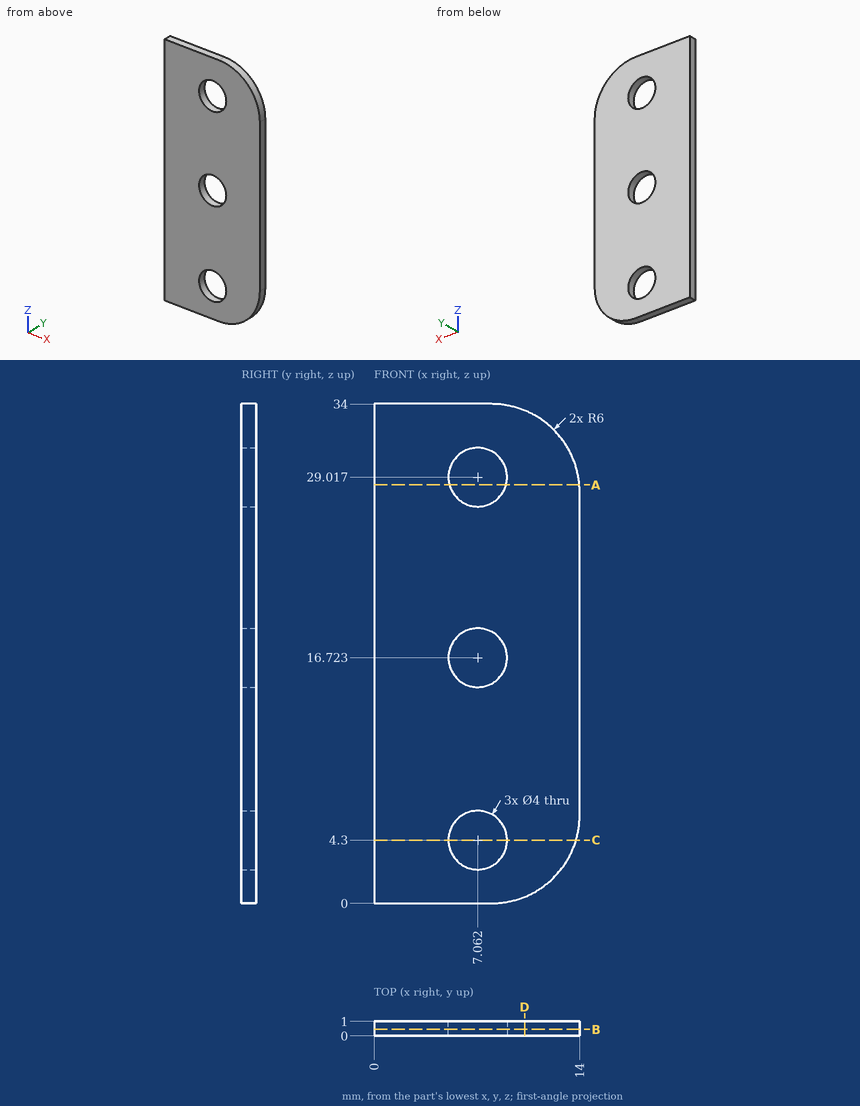
Drawing for the job (mm, zero at the part's lowest x, y, z). Round coordinates to 2 decimals unless told otherwise and drop trailing zeros. Loops run counter-clockwise (first coordinate to the right, second up) from the corner with the lowest first, then second, coordinate; pieces in that order, holes last.
1. Band-saw the part on B-B, the plane y = 0.45. List the corners of the cut face in (x, z), and give its area (3 significant figures).
Check values:
outline: (0, 0) - (8, 0) arc R6 ccw to (14, 6) - (14, 28) arc R6 ccw to (8, 34) - (0, 34) - close; hole circle Ø4 at (7.06, 4.3); hole circle Ø4 at (7.06, 16.72); hole circle Ø4 at (7.06, 29.02)
area: 423 mm2
2. Wall check: probe 1 along Z at (x, y) = (7, 0.8) (1 decimal); probe 2 along X at (y, z) = (0.7, 29) (1 decimal); probe 3 along X at (y, z) = (0.3, 18.5) (1 decimal). Give the ranges that are in metal, low to high.
Check values:
probe 1: z = 0 to 2.3, 6.3 to 14.7, 18.7 to 27, 31 to 34
probe 2: x = 0 to 5.1, 9.1 to 13.9
probe 3: x = 0 to 6.1, 8 to 14
3. Band-saw the part on D-D, the plane x = 10.25. List the corners of the cut face in (y, z).
Check values:
outline: (0, 0.44) - (1, 0.44) - (1, 33.56) - (0, 33.56) - close
4. Band-saw the part on A-A, the plane z = 28.5. List the corners of the cut face in (x, y), and give its area (3 significant figures).
Check values:
outline: (0, 0) - (5.13, 0) - (5.13, 1) - (0, 1) - close; (8.99, 0) - (13.98, 0) - (13.98, 1) - (8.99, 1) - close
area: 10.1 mm2
5. Band-saw the part on C-C, the plane z = 4.3. List the corners of the cut face in (x, y) (1 decimal).
Check values:
outline: (0, 0) - (5.1, 0) - (5.1, 1) - (0, 1) - close; (9.1, 0) - (13.8, 0) - (13.8, 1) - (9.1, 1) - close
